```python
from build123d import *

# Parameters (mm, degrees)
SKIZZE2_W                       = 8.6
SKIZZE2_H                       = 8.6
SKIZZE2_W_2                     = 8
SKIZZE2_H_2                     = 8
AUFSATZ_LINEAR_AUSTRAGEN1_DEPTH = 0.6
SKIZZE5_W                       = 8.6
SKIZZE5_H                       = 8.6
AUFSATZ_LINEAR_AUSTRAGEN3_DEPTH = 0.35
SKIZZE4_W                       = 8.6
SKIZZE4_H                       = 8.6
AUFSATZ_LINEAR_AUSTRAGEN2_DEPTH = 0.3
SKIZZE7_W                       = 8.6
SKIZZE7_H                       = 8.6
SKIZZE7_R                       = 2.8
AUFSATZ_LINEAR_AUSTRAGEN4_DEPTH = 1.8
SKIZZE8_R                       = 3.8
SKIZZE8_R_2                     = 2.8
AUFSATZ_LINEAR_AUSTRAGEN5_DEPTH = 0.9
FASE1_SIZE                      = 0.4


with BuildPart() as part:
    # Skizze2 → Aufsatz-Linear austragen1 (new body)
    with BuildSketch(Plane(origin=(0, 0, 0), x_dir=(1, 0, 0), z_dir=(0, 1, 0))):
        Rectangle(SKIZZE2_W, SKIZZE2_H)
        Rectangle(SKIZZE2_W_2, SKIZZE2_H_2, mode=Mode.SUBTRACT)
    extrude(amount=AUFSATZ_LINEAR_AUSTRAGEN1_DEPTH)

    # Skizze5 → Aufsatz-Linear austragen3 (add)
    with BuildSketch(Plane(origin=(0, 0.6, 0), x_dir=(1, 0, 0), z_dir=(0, 1, 0))):
        Rectangle(SKIZZE5_W, SKIZZE5_H)
        with BuildLine():
            Line((-2.764589803, 3.2), (2.764589803, 3.2))
            ThreePointArc((2.764589803, 3.2), (3.347487373, 3.347487373), (3.2, 2.764589803))
            Line((3.2, 2.764589803), (3.2, -2.764589803))
            ThreePointArc((3.2, -2.764589803), (3.347487373, -3.347487373), (2.764589803, -3.2))
            Line((2.764589803, -3.2), (-2.764589803, -3.2))
            ThreePointArc((-2.764589803, -3.2), (-3.347487373, -3.347487373), (-3.2, -2.764589803))
            Line((-3.2, -2.764589803), (-3.2, 2.764589803))
            ThreePointArc((-3.2, 2.764589803), (-3.347487373, 3.347487373), (-2.764589803, 3.2))
        make_face(mode=Mode.SUBTRACT)
    extrude(amount=AUFSATZ_LINEAR_AUSTRAGEN3_DEPTH)

    # Skizze4 → Aufsatz-Linear austragen2 (add)
    with BuildSketch(Plane(origin=(0, 0.95, 0), x_dir=(1, 0, 0), z_dir=(0, 1, 0))):
        Rectangle(SKIZZE4_W, SKIZZE4_H)
        with BuildLine():
            Line((-1.55, 2.15), (1.55, 2.15))
            ThreePointArc((1.55, 2.15), (1.974264069, 1.974264069), (2.15, 1.55))
            Line((2.15, 1.55), (2.15, -1.55))
            ThreePointArc((2.15, -1.55), (1.974264069, -1.974264069), (1.55, -2.15))
            Line((1.55, -2.15), (-1.55, -2.15))
            ThreePointArc((-1.55, -2.15), (-1.974264069, -1.974264069), (-2.15, -1.55))
            Line((-2.15, -1.55), (-2.15, 1.55))
            ThreePointArc((-2.15, 1.55), (-1.974264069, 1.974264069), (-1.55, 2.15))
        make_face(mode=Mode.SUBTRACT)
    extrude(amount=AUFSATZ_LINEAR_AUSTRAGEN2_DEPTH)

    # Skizze7 → Aufsatz-Linear austragen4 (add)
    with BuildSketch(Plane(origin=(0, 1.25, 0), x_dir=(1, 0, 0), z_dir=(0, 1, 0))):
        Rectangle(SKIZZE7_W, SKIZZE7_H)
        with Locations(Location((0, 0, 0), (0, 0, 270))):
            Circle(SKIZZE7_R, mode=Mode.SUBTRACT)
    extrude(amount=AUFSATZ_LINEAR_AUSTRAGEN4_DEPTH)

    # Skizze8 → Aufsatz-Linear austragen5 (add)
    with BuildSketch(Plane(origin=(0, 3.05, 0), x_dir=(1, 0, 0), z_dir=(0, 1, 0))):
        with Locations(Location((0, 0, 0), (0, 0, 270))):
            Circle(SKIZZE8_R)
        with Locations(Location((0, 0, 0), (0, 0, 270))):
            Circle(SKIZZE8_R_2, mode=Mode.SUBTRACT)
    extrude(amount=AUFSATZ_LINEAR_AUSTRAGEN5_DEPTH)

    # Fase1
    fase1_edges = [part.edges().sort_by_distance(p)[0] for p in [
        (0, 3.95, -2.8),
    ]]
    chamfer(fase1_edges, length=FASE1_SIZE)


solid = part.part
```
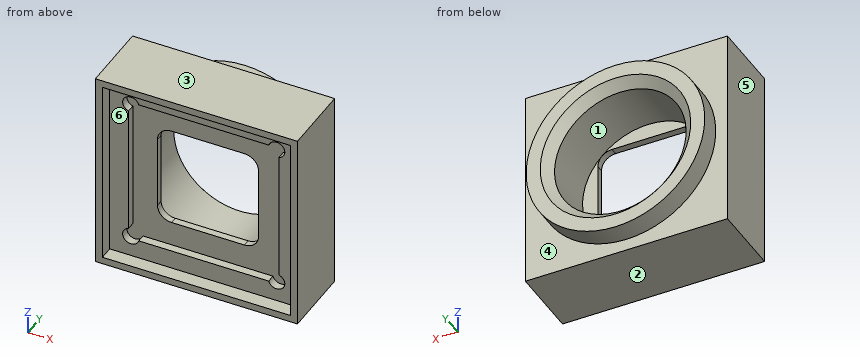
The listing builds one solid part. Answer for the finished solid, in the listing's coordinates (mm). Face numbers are marked on the shaded views. A direction names the side the tool comes from. Round coordinates to 2 decimals unless told otherwise and drop trailing zeros. Order: outer loops, then holes, each group sorted by start corner. A loop starts at its lowest first (then second) coordinate and runs counter-clockwise, first axis right, second up. Notation, with made-up numbers: (-13, 42.25) - (40, 42.25) arc R3 ccw to (40, 46.25) - close; hole circle Ø8 at (59.5, 50.25). An arc over 180 degrees is marked (long way). Put each result on its own line as item: value. Start each with the question number.
(1) Determine the mould class of the marked faces 1, 2 and 3 for opening direction Z: released by +Z, released by -Z, zero draft, split by the parting line, or undercut.
(2) Find section B-B (z = 0). Give the vertices of the cut face in (x, y), plus the area to 3 significant figures.
(3) Find section C-C (y = 3.2). Give the vertices of the cut face in (x, z), plus the area to 3 significant figures.
(4) For the marked faces 4, 5 and 6, determine the directions among +Z, -Z, +X, -X, +Y, -Y from which every point of the face is accessible in a straight line to the end or side of a thin tool.
(5) Find section A-A (x = 0). Give the vertices of the cut face in (y, z).
(6) Straight lines are drawn through the part: probe 1 along Z at (x, y) = (3.1, 0.85); probe 2 along X at (y, z) = (1, -1.5). For each, find the intervals that lie inside material, in ascending order. Write a range as from..to.
(7) Given P1, Ø1, axis at x = 3, z = 2.5, coming from the -Y side; P2, Ø1, axis at x = 1, z = 0.5, coming from the +Y side, each flat-ended and moving along its own axis, determine where each tip first touches the part or whether it passes through.
Reply:
1. face 1: undercut
1. face 2: released by -Z
1. face 3: released by +Z
2. outline: (-4.3, 0) - (-4, 0) - (-4, 0.6) - (-3.2, 0.6) - (-3.2, 0.95) - (-2.15, 0.95) - (-2.15, 1.25) - (-2.8, 1.25) - (-2.8, 3.55) - (-3.2, 3.95) - (-3.8, 3.95) - (-3.8, 3.05) - (-4.3, 3.05) - close; (2.15, 0.95) - (3.2, 0.95) - (3.2, 0.6) - (4, 0.6) - (4, 0) - (4.3, 0) - (4.3, 3.05) - (3.8, 3.05) - (3.8, 3.95) - (3.2, 3.95) - (2.8, 3.55) - (2.8, 1.25) - (2.15, 1.25) - close
2. area: 9.46 mm^2
3. outline: circle Ø7.6 at (0, 0); hole circle Ø5.6 at (0, 0)
3. area: 20.7 mm^2
4. face 4: +Y
4. face 5: +Z, -Z, -X, +Y, -Y
4. face 6: -Y
5. outline: (0, -4.3) - (3.05, -4.3) - (3.05, -3.8) - (3.95, -3.8) - (3.95, -3.2) - (3.55, -2.8) - (1.25, -2.8) - (1.25, -2.15) - (0.95, -2.15) - (0.95, -3.2) - (0.6, -3.2) - (0.6, -4) - (0, -4) - close; (0, 4) - (0.6, 4) - (0.6, 3.2) - (0.95, 3.2) - (0.95, 2.15) - (1.25, 2.15) - (1.25, 2.8) - (3.55, 2.8) - (3.95, 3.2) - (3.95, 3.8) - (3.05, 3.8) - (3.05, 4.3) - (0, 4.3) - close
6. probe 1: -4.3..-3.45, 3.45..4.3
6. probe 2: -4.3..-2.15, 2.15..4.3
7. P1: y = 0.6
7. P2: through
